```python
from build123d import *

# Parameters (mm, degrees)
BOSS_EXTRUDE1_DEPTH = 5
SKETCH_1_R          = 1.35
CUT_EXTRUDE_1_DEPTH = 30.045539702
SKETCH_2_R          = 4.265
SKETCH_2_R_2        = 2.265
EXTRUDE_1_DEPTH     = 3
EXTRUDE_2_DEPTH     = 5


with BuildPart() as part:
    # Sketch1 → Boss-Extrude1 (new body)
    with BuildSketch(Plane(origin=(0, 4, 0), x_dir=(1, 0, 0), z_dir=(0, 1, 0))):
        with BuildLine():
            ThreePointArc((-24.562186363, 2.217928037), (-24.606223651, 1.908945561), (-24.643657446, 1.599093719))
            ThreePointArc((-24.643657446, 1.599093719), (-23.481710119, 0.916420874), (-22.186907731, 0.542722358))
            ThreePointArc((-22.186907731, 0.542722358), (-12.402167869, -11.872817218), (1.305695063, -4))
            ThreePointArc((1.305695063, -4), (1.985007572, -0.183996455), (1.422120465, 3.650909885))
            ThreePointArc((1.422120465, 3.650909885), (1.757918397, 3.814049117), (2.081641936, 4))
            ThreePointArc((2.081641936, 4), (2.861028333, 4.588201733), (3.521749436, 5.30713988))
            ThreePointArc((3.521749436, 5.30713988), (3.405395609, 5.596745198), (3.282888305, 5.883801663))
            ThreePointArc((3.282888305, 5.883801663), (1.93527598, 5.894040025), (0.627094961, 5.57027124))
            ThreePointArc((0.627094961, 5.57027124), (0.366286148, 6.046375), (0.084372603, 6.510293938))
            ThreePointArc((0.084372603, 6.510293938), (1.018855105, 7.48132754), (1.683794586, 8.65351323))
            ThreePointArc((1.683794586, 8.65351323), (1.496450048, 8.903135899), (1.303821399, 9.148703928))
            ThreePointArc((1.303821399, 9.148703928), (-0.000522033, 8.809805691), (-1.180330337, 8.158486898))
            ThreePointArc((-1.180330337, 8.158486898), (-1.555477026, 8.550865528), (-1.947855656, 8.926012217))
            ThreePointArc((-1.947855656, 8.926012217), (-1.296536862, 10.105820521), (-0.957638625, 11.410163953))
            ThreePointArc((-0.957638625, 11.410163953), (-1.203206655, 11.602792602), (-1.452829324, 11.79013714))
            ThreePointArc((-1.452829324, 11.79013714), (-2.625015014, 11.125197659), (-3.596048616, 10.190715157))
            ThreePointArc((-3.596048616, 10.190715157), (-4.059967554, 10.472628702), (-4.536071314, 10.733437515))
            ThreePointArc((-4.536071314, 10.733437515), (-4.212302529, 12.041618533), (-4.222540891, 13.389230859))
            ThreePointArc((-4.222540891, 13.389230859), (-4.509597355, 13.511738163), (-4.799202674, 13.62809199))
            ThreePointArc((-4.799202674, 13.62809199), (-5.759348103, 12.682425791), (-6.455432668, 11.528463019))
            ThreePointArc((-6.455432668, 11.528463019), (-6.976508546, 11.680699536), (-7.503891752, 11.809396783))
            ThreePointArc((-7.503891752, 11.809396783), (-7.529737283, 13.156800143), (-7.888414517, 14.455843809))
            ThreePointArc((-7.888414517, 14.455843809), (-8.197396993, 14.499881098), (-8.507248835, 14.537314892))
            ThreePointArc((-8.507248835, 14.537314892), (-9.18992168, 13.375367565), (-9.563620196, 12.080565177))
            ThreePointArc((-9.563620196, 12.080565177), (-10.106342554, 12.09275), (-10.649064912, 12.080565177))
            ThreePointArc((-10.649064912, 12.080565177), (-11.022763428, 13.375367565), (-11.705436272, 14.537314892))
            ThreePointArc((-11.705436272, 14.537314892), (-12.015288115, 14.499881098), (-12.324270591, 14.455843809))
            ThreePointArc((-12.324270591, 14.455843809), (-12.682947825, 13.156800143), (-12.708793355, 11.809396783))
            ThreePointArc((-12.708793355, 11.809396783), (-13.236176561, 11.680699536), (-13.757252439, 11.528463019))
            ThreePointArc((-13.757252439, 11.528463019), (-14.453337005, 12.682425791), (-15.413482434, 13.62809199))
            ThreePointArc((-15.413482434, 13.62809199), (-15.703087752, 13.511738163), (-15.990144217, 13.389230859))
            ThreePointArc((-15.990144217, 13.389230859), (-16.000382579, 12.041618533), (-15.676613793, 10.733437515))
            ThreePointArc((-15.676613793, 10.733437515), (-16.152717554, 10.472628702), (-16.616636492, 10.190715157))
            ThreePointArc((-16.616636492, 10.190715157), (-17.587670094, 11.125197659), (-18.759855783, 11.79013714))
            ThreePointArc((-18.759855783, 11.79013714), (-19.009478453, 11.602792602), (-19.255046482, 11.410163953))
            ThreePointArc((-19.255046482, 11.410163953), (-18.916148245, 10.105820521), (-18.264829452, 8.926012217))
            ThreePointArc((-18.264829452, 8.926012217), (-18.657208082, 8.550865528), (-19.032354771, 8.158486898))
            ThreePointArc((-19.032354771, 8.158486898), (-20.212163074, 8.809805691), (-21.516506507, 9.148703928))
            ThreePointArc((-21.516506507, 9.148703928), (-21.709135156, 8.903135899), (-21.896479694, 8.65351323))
            ThreePointArc((-21.896479694, 8.65351323), (-21.231540213, 7.48132754), (-20.297057711, 6.510293938))
            ThreePointArc((-20.297057711, 6.510293938), (-20.578971255, 6.046375), (-20.839780068, 5.57027124))
            ThreePointArc((-20.839780068, 5.57027124), (-22.147961087, 5.894040025), (-23.495573413, 5.883801663))
            ThreePointArc((-23.495573413, 5.883801663), (-23.618080717, 5.596745198), (-23.734434544, 5.30713988))
            ThreePointArc((-23.734434544, 5.30713988), (-22.788768345, 4.346994451), (-21.634805572, 3.650909885))
            ThreePointArc((-21.634805572, 3.650909885), (-21.78704209, 3.129834008), (-21.915739337, 2.602450802))
            ThreePointArc((-21.915739337, 2.602450802), (-23.263142697, 2.576605271), (-24.562186363, 2.217928037))
        make_face()
    extrude(amount=-BOSS_EXTRUDE1_DEPTH)

    # 草图1 → 切除-拉伸1 (cut, through all)
    with BuildSketch(Plane.XZ.offset(1)):
        with Locations(Location((-10.106342554, 0, 0), (0, 0, 270))):
            Circle(SKETCH_1_R)
    extrude(amount=-CUT_EXTRUDE_1_DEPTH, mode=Mode.SUBTRACT)

    # 草图2 → 凸台-拉伸1 (add)
    with BuildSketch(Plane.XZ.offset(1)):
        with Locations(Location((-10.106342554, 0, 0), (0, 0, 90))):
            Circle(SKETCH_2_R)
        with Locations(Location((-10.106342554, 0, 0), (0, 0, 270))):
            Circle(SKETCH_2_R_2, mode=Mode.SUBTRACT)
    extrude(amount=EXTRUDE_1_DEPTH)

    # 草图3 → 凸台-拉伸2 (add)
    with BuildSketch(Plane.XZ.offset(1)):
        with BuildLine():
            Line((1.316832407, 9.59169813), (-1.732440783, 8.724240465))
            Line((-1.732440783, 8.724240465), (1.660979616, -2.786526782))
            Line((1.660979616, -2.786526782), (10.317511543, -0.323915364))
            ThreePointArc((10.317511543, -0.323915364), (23.060971172, 14.056333138), (41.465450985, 8.537054824))
            Line((41.465450985, 8.537054824), (53.333346557, 11.913235424))
            ThreePointArc((53.333346557, 11.913235424), (26.628358933, 26.363456331), (1.316832407, 9.59169813))
        make_face()
    extrude(amount=-EXTRUDE_2_DEPTH)

    # 草图5 → 切除-旋转1 (revolve, cut)
    with BuildSketch(Plane(origin=(8.606089679, 0, -14.547237495), x_dir=(-0.8606674274779063, 0, -0.5091675355701334), z_dir=(0.5091675355701334, 0, -0.8606674274779063))):
        Polygon((-43.768106901, 4), (-39.968106901, -1.23415978), (-39.968106901, 4), align=None)
    revolve(axis=Axis((27.943657446, -0.047851862, -3.107206875), (0, -1, 0)), mode=Mode.SUBTRACT)


solid = part.part
```
Could you check a few things on this model? Use its own coordinates, in mm. A direction names the side the tool comes from. Give positions to 0.01 mm unless a question says otherwise; leave off trailing zeros. Write each loop counter-clockwise with the first axis right and the second up, starting at its lowest first coordinate (ties: lowest second). Pieces come first, ordered by that corner, then holes. Notation, with made-up numbers: (63, -6) - (110, -6) arc R27 cw to (110, 32) - close; hole circle Ø11 at (-39, 66.5). An arc over 180 degrees is marked (long way). One line per item, written item: value. Start each with the question number.
Item 1: Which directions (+Z, -Z, +X, -X, +Y, -Y) give clear straight access to the entire face, cutting with the end or side of a thin tool? Please do faces 1 (the face through (-12.317, -2.479, 0.491)), 2 (the face through (-11.015, 1.535, -13.358)), 3 (the face through (1.01, 1.54, -7.47)), 4 (the face through (-22.13, 1.54, -5.89)).
Item 2: Please list where these lines run through material, in increasing order: line 1 (X direction, y = -2.8, z = 0); line 2 (Y direction, x = -6, z = 6.5); line 3 (X direction, y = 1.95, z = 0). Write a range as from..to.
Item 3: I'm going to push flat-ended pins straight in: pin 1 (2 mm diameter, centred on y = -1, z = -6, fed in from -X); pin 2 (3 mm diameter, centred on x = -10.11, z = 0, fed in from -Y); pin 3 (1 mm diameter, centred on y = 2.5, z = 21, fed in from -X). Where does each tip first touch, or does it pass through?
Item 4: If we mould it in two halves opening along Z, with no side actions, what happens to faces 5 (the face through (-1.3, 1.5, -10.1)), 6 (the face through (-22.804, 1.535, -4.359)), 7 (the face through (-14.442, 1.535, -12.668)), 8 (the face through (27.07, 1.46, 26.38))? For each: +Z half, -Z half, draft (parallel to the pull), parting line (faces both ways), or undercut.
Item 5: Imagine slicing it at A-A, the plane y = -2.25. List the corners of the cut face in (x, z) for me (3 decimals), and give its area (3 significant figures).
Geometry says:
1. face 1: -Y
1. face 2: -Z, +Y, -Y
1. face 3: +X, +Y, -Y
1. face 4: +Y, -Y
2. line 1: -14.37..-12.37, -7.84..-5.84
2. line 2: -1..4
2. line 3: -22.2..-11.46, -8.76..8.38
3. pin 1: x = -23.73
3. pin 2: y = -1
3. pin 3: x = 10.25
4. face 5: undercut
4. face 6: undercut
4. face 7: -Z half
4. face 8: +Z half
5. outline: circle Ø8.53 at (-10.106, 0); hole circle Ø4.53 at (-10.106, 0)
5. area: 41.0 mm^2
